Input: part model. Units: mm. Frame: model coordinates. A direction names the side the tool comes from. Coordinates: 2 decimals unless noted, no trailing zeros. Order: outer loops, then holes, each group sorted by start corner. A loop starts at its lowest first (then second) coordinate and runs counter-clockwise, first axis right, second up. Notation, with made-up numbers: (-9, -39.5) -> (21, -39.5) arc R19 ccw to (21, -29.5) -> close; hole circle Ø1 at (5.25, 75). An arc over 180 degrees is marked (long way). One line per question, with ' | ' between items.
```python
from build123d import *

# Parameters (mm, degrees)
MODEL_W             = 5.350000225
MODEL_H             = 20.000001416
MODEL_W_2           = 5.349997431
MODEL_W_3           = 11.000000872
MODEL_H_2           = 5.350001156
MODEL_H_3           = 19.999999553
MODEL_H_4           = 20.000003278
MODEL_W_4           = 13.99999857
MODEL_H_5           = 5.350008607
MODEL_W_5           = 14.000000433
MODEL_W_6           = 13.999999967
MODEL_H_6           = 5.350000225
MODEL_W_7           = 4.999999888
MODEL_H_7           = 5.349997431
MODEL_W_8           = 4.999998957
MODEL_W_9           = 5.000002682
BOSS_EXTRUDE1_DEPTH = 5.35


with BuildPart() as part:
    # Model → Boss-Extrude1 (new body)
    with BuildSketch(Plane.XY):
        with BuildLine():
            Line((4.000000656, 29.99999933), (19.694138318, 29.99999933))
            ThreePointArc((19.694138318, 29.99999933), (21.815457776, 30.878679471), (22.694136947, 32.999999329))
            Line((22.694136947, 32.999999329), (22.694136947, 199.99999553))
            Line((22.694136947, 199.99999553), (92.694137245, 199.99999553))
            Line((92.694137245, 199.99999553), (92.694137245, 32.999999821))
            ThreePointArc((92.694137245, 32.999999821), (93.572816728, 30.87867916), (95.694137245, 29.99999933))
            Line((95.694137245, 29.99999933), (111.388277918, 29.99999933))
            ThreePointArc((111.388277918, 29.99999933), (114.216704616, 28.828426881), (115.388277918, 26.000000537))
            Line((115.388277918, 26.000000537), (115.388277918, 4))
            ThreePointArc((115.388277918, 4), (114.216704811, 1.171572643), (111.388277262, 0))
            Line((111.388277262, 0), (4, 0))
            ThreePointArc((4, 0), (1.171572643, 1.171573107), (0, 4.000000656))
            Line((0, 4.000000656), (0, 25.99999933))
            ThreePointArc((0, 25.99999933), (1.171573107, 28.828426686), (4.000000656, 29.99999933))
        make_face()
        with Locations((84.849137348, 82.500000484)):
            Rectangle(MODEL_W, MODEL_H, mode=Mode.SUBTRACT)
        with Locations((30.539138243, 82.500000484)):
            Rectangle(MODEL_W_2, MODEL_H, mode=Mode.SUBTRACT)
        with Locations((57.694137562, 104.249998927)):
            Rectangle(MODEL_W_3, MODEL_H_2, mode=Mode.SUBTRACT)
        with Locations((84.849137348, 124.999998138)):
            Rectangle(MODEL_W, MODEL_H_3, mode=Mode.SUBTRACT)
        with Locations((30.539138243, 124.999998138)):
            Rectangle(MODEL_W_2, MODEL_H_3, mode=Mode.SUBTRACT)
        with Locations((30.539138243, 167.500000447)):
            Rectangle(MODEL_W_2, MODEL_H_4, mode=Mode.SUBTRACT)
        with Locations((84.849137348, 167.500000447)):
            Rectangle(MODEL_W, MODEL_H_4, mode=Mode.SUBTRACT)
        with Locations((57.694137562, 145.749997348)):
            Rectangle(MODEL_W_3, MODEL_H_2, mode=Mode.SUBTRACT)
        with Locations((43.694138527, 189.824998379)):
            Rectangle(MODEL_W_4, MODEL_H_5, mode=Mode.SUBTRACT)
        with Locations((71.694137529, 189.824998379)):
            Rectangle(MODEL_W_5, MODEL_H_5, mode=Mode.SUBTRACT)
        with Locations((71.444137721, 42.024999392)):
            Rectangle(MODEL_W_6, MODEL_H_6, mode=Mode.SUBTRACT)
        with Locations((43.44413802, 42.024999392)):
            Rectangle(MODEL_W_4, MODEL_H_6, mode=Mode.SUBTRACT)
        with Locations((85.869137663, 10.22499986)):
            Rectangle(MODEL_W_7, MODEL_H_7, mode=Mode.SUBTRACT)
        with Locations((110.869137571, 10.22499986)):
            Rectangle(MODEL_W_8, MODEL_H_7, mode=Mode.SUBTRACT)
        with Locations((4.519138485, 10.22499986)):
            Rectangle(MODEL_W_9, MODEL_H_7, mode=Mode.SUBTRACT)
        with Locations((29.519138858, 10.22499986)):
            Rectangle(MODEL_W_8, MODEL_H_7, mode=Mode.SUBTRACT)
        with BuildLine():
            Line((12.999996543, 17.000000924), (5.000000656, 17.000000924))
            ThreePointArc((5.000000656, 17.000000924), (4.292894475, 17.292893542), (4.000000656, 17.999999225))
            Line((4.000000656, 17.999999225), (4.000000656, 25.000000537))
            ThreePointArc((4.000000656, 25.000000537), (4.292891957, 25.7071054), (4.999995232, 26.000000536))
            Line((4.999995232, 26.000000536), (12.99999857, 26.000000536))
            ThreePointArc((12.99999857, 26.000000536), (13.707106067, 25.707106601), (13.99999857, 24.99999851))
            Line((13.99999857, 24.99999851), (13.99999857, 18.000000924))
            ThreePointArc((13.99999857, 18.000000924), (13.707104634, 17.292893426), (12.999996543, 17.000000924))
        make_face(mode=Mode.SUBTRACT)
    extrude(amount=BOSS_EXTRUDE1_DEPTH)


solid = part.part
```
1. Cut plane B-B, the plane y = 86. Return loops of the section in (x, z).
Recorded:
outline: (22.69, 0) -> (27.86, 0) -> (27.86, 5.35) -> (22.69, 5.35) -> close; (33.21, 0) -> (82.17, 0) -> (82.17, 5.35) -> (33.21, 5.35) -> close; (87.52, 0) -> (92.69, 0) -> (92.69, 5.35) -> (87.52, 5.35) -> close
2. Cut plane D-D, the plane y = 60.5. Return loops of the section in (x, z), and give its area (4 significant figures).
Recorded:
outline: (22.69, 0) -> (92.69, 0) -> (92.69, 5.35) -> (22.69, 5.35) -> close | area: 374.5 mm^2
3. Mould query, pull axis Y, two halves, no side actions, for faces 1 (the face through (12, 30, 3)), 2 (the face through (36.694, 190, 3)), 3 (the face through (58, 0, 3)), 4 (the face through (59, 79, 5.35)). Classes: released by +Y, released by -Y, zero draft, split by the parting line, or undercut.
Recorded:
face 1: released by +Y | face 2: undercut | face 3: released by -Y | face 4: zero draft
4. Cut plane A-A, the plane x = 47. Return loops of the section in (y, z), and give its area (3 significant figures).
Recorded:
outline: (0, 0) -> (39.35, 0) -> (39.35, 5.35) -> (0, 5.35) -> close; (44.7, 0) -> (187.15, 0) -> (187.15, 5.35) -> (44.7, 5.35) -> close; (192.5, 0) -> (200, 0) -> (200, 5.35) -> (192.5, 5.35) -> close | area: 1,010 mm^2
5. Ray query, line 1 (X direction, y = 190.5, z = 2.8); line 2 (Y direction, x = 40.5, z = 3.2); line 3 (X direction, y = 132, z = 3.5). Return the intervals inside material, ascending. Write a range as [from, to].
Recorded:
line 1: x = [22.69, 36.69], [50.69, 64.69], [78.69, 92.69] | line 2: y = [0, 39.35], [44.7, 187.15], [192.5, 200] | line 3: x = [22.69, 27.86], [33.21, 82.17], [87.52, 92.69]
6. Pin query (flat end, axial travel): pin 1 Ø3 at (y, z) = (35, 1) entering from +X; pin 2 Ø1 at (y, z) = (164, 2.5) entering from -X; pin 3 Ø6 at (x, y) = (22.5, 71.5) entering from -Z. Return the tip coordinate at first contact, or that it passes through.
Recorded:
pin 1: stops at x = 92.69 | pin 2: stops at x = 22.69 | pin 3: stops at z = 0
7. Cut plane C-C, the plane z = 2.25. State how many separate pieces and enclosed holes the cut face has, and give its area (3 significant figures).
Recorded:
separate pieces: 1 | enclosed holes: 17 | area: 14,100 mm^2
8. Access query for faces 5 (the face through (103, 30, 3)), 6 (the face through (59, 79, 0)), 7 (the face through (85, 115, 3)). Directions: +Z, -Z, +X, -X, +Y, -Y. A direction counts if a zero-diameter tool reaches every point of the face in a straight line with its end or side. Return the directions, or none.
Recorded:
face 5: +Z, -Z, +X, +Y | face 6: -Z, +X, -X, +Y, -Y | face 7: +Z, -Z
